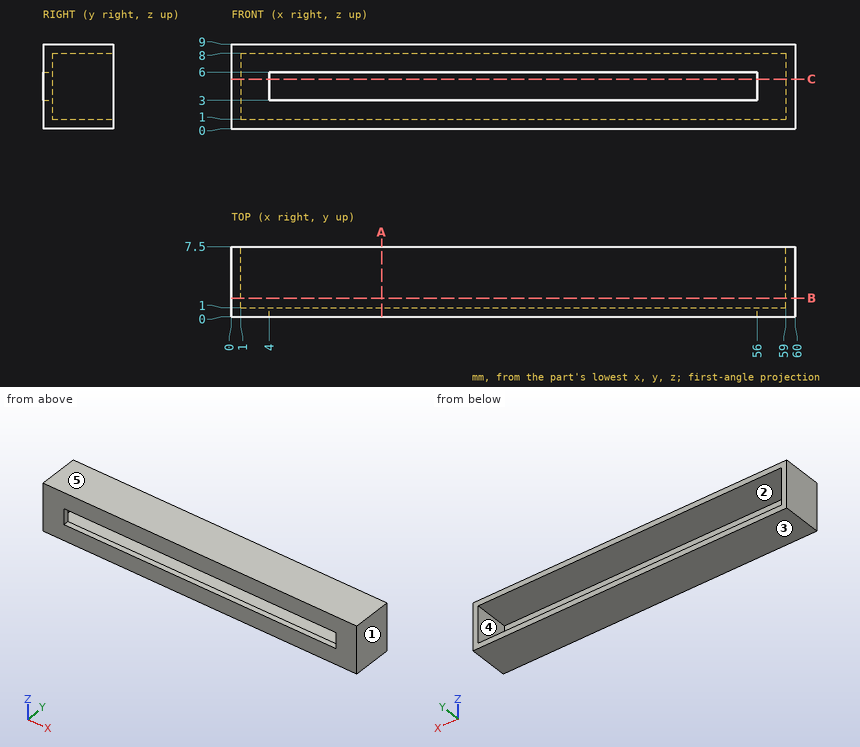
Design review of the part shown in the three views and the two pictorial views. Dimensions are in mm from the part's minimum x, y and z. A direction names the side the tool comes from. Give positions to 0.01 mm unless a question says otherwise; leave off trailing zeros. Write each loop counter-clockwise with the first axis right and the second up, starting at its lowest first coordinate (ties: lowest second). Pieces come first, ordered by that corner, then holes.
Item 1: Machinability: for the marked faces 1 and 2, which of the approach directions +Z, -Z, +X, -X, +Y, -Y give a long, thin tool a straight path to every point of the face, cutting with its end or side? Answer none if there is none.
Item 2: Wall thickness on probe 1 along X at (y, z) = (1.25, 5); probe 2 along Z at (x, y) = (16.5, 1.5); probe 3 along X at (y, z) = (0.5, 4.75): over which ranges is each line inside the solid? List them lowest first.
Item 3: Insertion check: P1, Ø2, axis at x = 39.5, z = 3.5, coming from the +Y side. The pin has a flat end and moves straight along its axis. Give the tip position at first contact, or say it passes through.
Item 4: The part is to be moulded in two halves that separate along Z. For the marked faces 3, 4 and 5, say which applies: +Z half, -Z half, draft (parallel to the pull), parting line (faces both ways), or undercut.
Item 5: Take a section at C-C (z = 5.25). Give the boundary of the cut face in (x, y).
Item 6: Take a section at A-A (x = 16). Give the boundary of the cut face in (y, z).
Item 7: Take a section at B-B (y = 2). Give the boundary of the cut face in (x, z).
Established:
1. face 1: +Z, -Z, +X, +Y, -Y
1. face 2: +Y
2. probe 1: x = 0 to 1, 59 to 60
2. probe 2: z = 0 to 1, 8 to 9
2. probe 3: x = 0 to 4, 56 to 60
3. P1: stops at y = 1
4. face 3: -Z half
4. face 4: undercut
4. face 5: +Z half
5. outline: (0, 0) - (4, 0) - (4, 1) - (1, 1) - (1, 7.5) - (0, 7.5) - close; (56, 0) - (60, 0) - (60, 7.5) - (59, 7.5) - (59, 1) - (56, 1) - close
6. outline: (0, 0) - (7.5, 0) - (7.5, 1) - (1, 1) - (1, 3) - (0, 3) - close; (0, 6) - (1, 6) - (1, 8) - (7.5, 8) - (7.5, 9) - (0, 9) - close
7. outline: (0, 0) - (60, 0) - (60, 9) - (0, 9) - close; hole (1, 1) - (59, 1) - (59, 8) - (1, 8) - close
